```python
from build123d import *

# Parameters (mm, degrees)
F0_R            = 10
F1_DEPTH        = 8.5
F3_DEPTH        = 5
F3_COPIES_COUNT = 20
F5_R            = 10
F6_DEPTH        = 0.9
F7_R            = 6
F8_DEPTH        = 0.3
F9_R            = 2.5
F10_DEPTH       = 14.7
F11_R           = 1.5
F12_REACH       = 14.2436406871


# Not quite as in the source:
# - a pattern or mirror of a feature is missing from the dataset's text; its kind, count and spacing are read off the source's solid


with BuildPart() as f1:
    # F0 (on Right) → F1 (new body)
    with BuildSketch(Plane.YZ):
        Circle(F0_R)
    extrude(amount=F1_DEPTH)

    # F2 (on face) → F3 (join)
    with BuildSketch(Plane.YZ.offset(8.5)):
        with BuildLine():
            Line((0.5, 6.4807406984), (0.5, 7.25))
            ThreePointArc((0.5, 7.25), (0, 7.75), (-0.5, 7.25))
            Line((-0.5, 7.25), (-0.5, 6.4807406984))
            ThreePointArc((-0.5, 6.4807406984), (0, -6.5), (0.5, 6.4807406984))
        make_face()
    f3 = extrude(amount=F3_DEPTH)

    # F3_copies: F3 ×20 about axis
    f3_copies_axis = Axis((0, 0, 0), (1, 0, 0))
    for i in range(1, F3_COPIES_COUNT):
        add(f3.rotate(f3_copies_axis, i * 360 / F3_COPIES_COUNT))

    # F5 (on face) → F6 (join)
    with BuildSketch(Plane.YZ.offset(13.5)):
        Circle(F5_R)
    extrude(amount=F6_DEPTH)

    # F7 (on face) → F8 (join)
    with BuildSketch(Plane.YZ.offset(14.4)):
        Circle(F7_R)
    extrude(amount=F8_DEPTH)

    # F9 (on face) → F10 (cut, through all)
    with BuildSketch(Plane.YZ.offset(14.7)):
        Circle(F9_R)
    extrude(amount=-F10_DEPTH, mode=Mode.SUBTRACT)

    f12_end = f1.faces().sort_by_distance((4.25, -10, 0))[0]
    # F11 (on Top) → F12 (cut, up to a face of the model that its end follows)
    with BuildSketch(Plane.XY):
        with Locations((4, 0)):
            Circle(F11_R)
    f12_long = extrude(amount=F12_REACH, mode=Mode.PRIVATE)
    add(split(f12_long, bisect_by=f12_end, keep=Keep.BOTTOM, mode=Mode.PRIVATE), mode=Mode.SUBTRACT)


solid = f1.part
```
Could you check a few things on this model? Use its own coordinates, in mm. A direction names the side the tool comes from. Coordinates: 2 decimals unless noted, no trailing zeros. Write each loop counter-clockwise with the first axis right and the second up, starting at its lowest first coordinate (ties: lowest second). Pieces come first, ordered by that corner, then holes. Notation, with made-up numbers: M 73.5,10 L 88.5,10 A15 cw 88.5,16 Z; hole C 20,33 d11. An arc over 180 degrees is marked long. Answer as CSV lines item,"result". Start each with the question number.
1) I want a section at C-C, the plane x = 6. Please give me the cut outline in (y, z), and give its area (3 significant figures).
2) Please list where these lines run through material, in increasing order: line 1 (Z direction, x = 11, y = 0); line 2 (X direction, y = 9.25, z = -1.75); line 3 (X direction, y = 0, z = 3.75). Write a range as from..to.
3) I want a section at D-D, the plane x = 4. Please give me the cut outline in (y, z), and give its area (3 significant figures).
4) For P1, Ø0.6, axis at x = 10.5, y = 7, coming from the +Z side; P2, Ø1.8, axis at x = 4, y = 0, coming from the +Z side; P3, Ø3, axis at y = 0, z = 0, coming from the +X side; P4, Ø4, axis at x = 1.5, y = -3.5, coming from the +Z side, each with a flat end and sliding along its axis, tell me the tip position at first contact or that it passes through.
5) I want a section at A-A, the plane y = 0. Please give me the cut outline in (x, z), and give its area (3 significant figures).
6) I want a section at B-B, the plane z = 0. Please give me the cut outline in (x, y), and give its area (3 significant figures).
7) For faces 1 (the cylindrical face through (10.965, -2.944, 5.795)), 2 (the cylindrical face through (10.96, -6.42, -1.01)), 3 (the cylindrical face through (10.96, 6.42, 1.01)), 4 (the cylindrical face through (10.96, 1.02, 6.42)), which set-ups out of +Z, -Z, +X, -X, +Y, -Y let a thin tool reach every point of the face, with its end or its side?
8) We'd pull the mould along Z, two halves only. Please class faces 5 (the cylindrical face through (10.965, 7.374, 2.384)), 6 (the flat face through (14.4, 0, -7)), 7 (the cylindrical face through (10.96, -1.02, -6.42)), 8 (the cylindrical face through (10.965, 4.564, 6.263)): +Z half, -Z half, draft (parallel to the pull), parting line (faces both ways), or undercut.
Data:
1,outline,"C 0,0 d20; hole C 0,0 d5"
1,area,"295 mm^2"
2,line 1,"z = -7.75..-2.5, 2.5..7.75"
2,line 2,"x = 0..8.5, 13.5..14.4"
2,line 3,"x = 0..2.5, 5.5..14.7"
3,outline,"M -1.5,2 L -1.5,9.89 A10 ccw long 1.5,9.89 L 1.5,2 A2.5 cw long Z"
3,area,"272 mm^2"
4,P1,"stops at z = 2.74"
4,P2,"stops at z = -2.33"
4,P3,"passes through"
4,P4,"stops at z = 9.89"
5,outline,"M 0,-10 L 8.5,-10 L 8.5,-7.75 L 13.5,-7.75 L 13.5,-10 L 14.4,-10 L 14.4,-6 L 14.7,-6 L 14.7,-2.5 L 0,-2.5 Z; M 0,2.5 L 2.5,2.5 L 2.5,10 L 0,10 Z; M 5.5,2.5 L 14.7,2.5 L 14.7,6 L 14.4,6 L 14.4,10 L 13.5,10 L 13.5,7.75 L 8.5,7.75 L 8.5,10 L 5.5,10 Z"
5,area,"173 mm^2"
6,outline,"M 0,-10 L 8.5,-10 L 8.5,-7.75 L 13.5,-7.75 L 13.5,-10 L 14.4,-10 L 14.4,-6 L 14.7,-6 L 14.7,-2.5 L 0,-2.5 Z; M 0,2.5 L 14.7,2.5 L 14.7,6 L 14.4,6 L 14.4,10 L 13.5,10 L 13.5,7.75 L 8.5,7.75 L 8.5,10 L 0,10 Z"
6,area,"196 mm^2"
7,face 1,"none"
7,face 2,"-Y"
7,face 3,"+Y"
7,face 4,"+Z"
8,face 5,"undercut"
8,face 6,"draft"
8,face 7,"-Z half"
8,face 8,"undercut"
